Here's how the part is built. I have some questions about the finished solid (model axes, mm). Face numbers are marked on the shaded views. A direction names the side the tool comes from. Round coordinates to 2 decimals unless told otherwise and drop trailing zeros. Write each loop counter-clockwise with the first axis right and the second up, starting at its lowest first coordinate (ties: lowest second). Pieces come first, ordered by that corner, then holes. Notation, with made-up numbers: (56.25, 33) - (89.25, 33) arc R23 ccw to (89.25, 58) - close; hole circle Ø8 at (46, -8). An arc over 180 degrees is marked (long way). Use one line per item in the form item = value. Start each with the question number.
1. I want a section at D-D, the plane z = 61.5. List the corners of the cut face in (x, y) for me.
2. Which directions (+Z, -Z, +X, -X, +Y, -Y) give clear straight access to the entire face, cutting with the end or side of a thin tool? Please do the marked faces 1 and 2.
3. We'd pull the mould along Y, two halves only. Please class the marked faces 3, 4 and 5: +Y half, -Y half, draft (parallel to the pull), parting line (faces both ways), or undercut.
4. I want a section at C-C, the plane y = -76.2. List the corners of the cut face in (x, z) for me.
5. I want a section at B-B, the plane x = 101.6. List the corners of the cut face in (y, z) for me.
6. If I drill on line 1 along Y through (x, z) = (101.6, 81.5); line 2 along X through (y, z) = (-110, 6.5); line 3 along Z through (x, y) = (87, -25.5), over which ranges is the centre line in solid material (lowest first)?
7. Will these pins go through, and if not, where does the flat tip stop? pin 1 (10 mm diameter, centred on y = -121.5, z = 21, fed in from -X); pin 2 (6 mm diameter, centred on x = 75.5, y = -86, fed in from -Z).
8. I want a section at A-A, the plane z = 44. List the corners of the cut face in (x, y) for me.
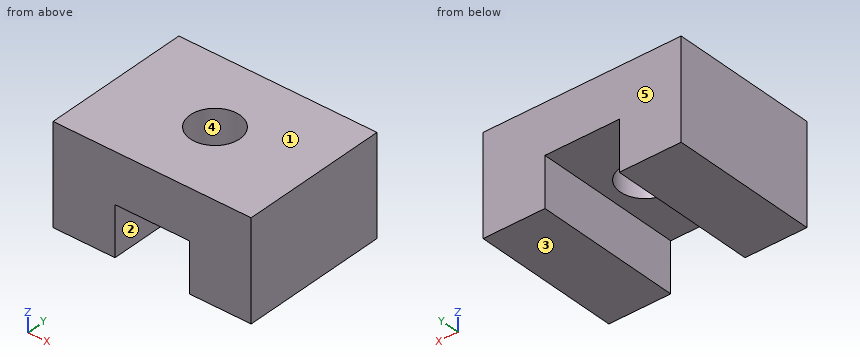
```python
from build123d import *

# Parameters (mm, degrees)
F1_DEPTH = 152.4
F2_R     = 25.4
F3_DEPTH = 101.601


with BuildPart() as f1:
    # F0 (on Front) → F1 (new body)
    with BuildSketch(Plane.XZ):
        Polygon((0, 101.6), (0, 0), (63.5, 0), (63.5, 50.8), (139.7, 50.8), (139.7, 0), (203.2, 0), (203.2, 101.6), align=None)
    extrude(amount=F1_DEPTH)

    # F2 (on face) → F3 (cut, through all)
    with BuildSketch(Plane.XY.offset(101.6)):
        with Locations((101.6, -76.2)):
            Circle(F2_R)
    extrude(amount=-F3_DEPTH, mode=Mode.SUBTRACT)


solid = f1.part
```
Model answer:
q1.outline = (0, -152.4) - (203.2, -152.4) - (203.2, 0) - (0, 0) - close; hole circle Ø50.8 at (101.6, -76.2)
q2.face_1 = +Z, +X, -X, +Y, -Y
q2.face_2 = -Z, +Y, -Y
q3.face_3 = draft
q3.face_4 = undercut
q3.face_5 = +Y half
q4.outline = (0, 0) - (63.5, 0) - (63.5, 50.8) - (76.2, 50.8) - (76.2, 101.6) - (0, 101.6) - close; (127, 50.8) - (139.7, 50.8) - (139.7, 0) - (203.2, 0) - (203.2, 101.6) - (127, 101.6) - close
q5.outline = (-152.4, 50.8) - (-101.6, 50.8) - (-101.6, 101.6) - (-152.4, 101.6) - close; (-50.8, 50.8) - (0, 50.8) - (0, 101.6) - (-50.8, 101.6) - close
q6.line_1 = -152.4 to -101.6, -50.8 to 0
q6.line_2 = 0 to 63.5, 139.7 to 203.2
q6.line_3 = 50.8 to 101.6
q7.pin_1 = 0
q7.pin_2 = 50.8
q8.outline = (0, -152.4) - (63.5, -152.4) - (63.5, 0) - (0, 0) - close; (139.7, -152.4) - (203.2, -152.4) - (203.2, 0) - (139.7, 0) - close
